CAD build for the part. Positions are in the model's coordinates, mm. Face numbers are marked on the shaded views. A direction names the side the tool comes from. Give positions to 0.01 mm unless a question says otherwise; leave off trailing zeros. Loops run counter-clockwise (first coordinate to the right, second up) from the corner with the lowest first, then second, coordinate; pieces in that order, holes last. Notation, with made-up numbers: M 72.25,47 L 88.25,47 A18 ccw 88.25,58 Z; hole C 73.25,42 d8. An arc over 180 degrees is marked long. One line per question, with ' | ' between items.
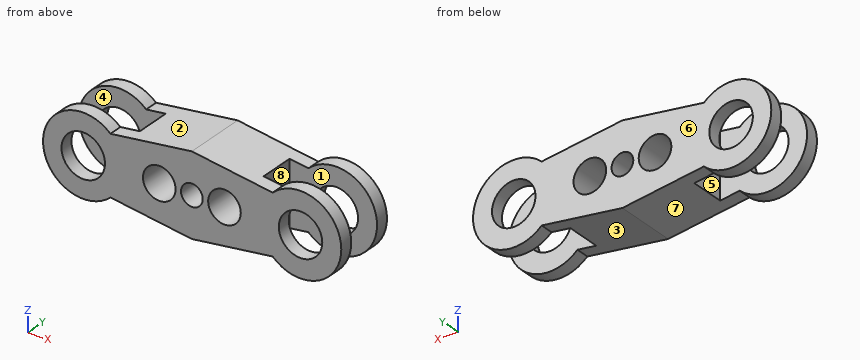
```python
from build123d import *

# Parameters (mm, degrees)
Y_KSEKLIK_EKSTR_ZYON1_OUTLINE_R   = 4
Y_KSEKLIK_EKSTR_ZYON1_OUTLINE_R_2 = 3
Y_KSEKLIK_EKSTR_ZYON1_OUTLINE_R_3 = 2
Y_KSEKLIK_EKSTR_ZYON1_DEPTH       = 11.5
KES_EKSTR_ZYON9_DEPTH             = 50
KES_EKSTR_ZYON9_DEPTH_BACK        = 50
IZIM16_W                          = 16
IZIM16_H                          = 6.5
IZIM16_W_2                        = 1.702500787


# Read off the part's stored shape, not the designer's step: Y_kseklik-Ekstr_zyon1
with BuildPart() as part:
    # Y_kseklik-Ekstr_zyon1 outline → Y_kseklik-Ekstr_zyon1 (new body)
    with BuildSketch(Plane(origin=(0, 0, 0), x_dir=(1, 0, 0), z_dir=(0, 1, 0))):
        with BuildLine():
            Line((-14.995122872, -5.45), (0, -7.5))
            Line((0, -7.5), (14.866270364, -5.46761557))
            ThreePointArc((14.866270364, -5.46761557), (27.5, 0), (14.866270364, 5.46761557))
            Line((14.866270364, 5.46761557), (0, 7.5))
            Line((0, 7.5), (-14.995122872, 5.45))
            ThreePointArc((-14.995122872, 5.45), (-27.399411806, 0), (-14.995122872, -5.45))
        make_face()
        with Locations((-20, 0)):
            Circle(Y_KSEKLIK_EKSTR_ZYON1_OUTLINE_R, mode=Mode.SUBTRACT)
        with Locations((-6, 0)):
            Circle(Y_KSEKLIK_EKSTR_ZYON1_OUTLINE_R_2, mode=Mode.SUBTRACT)
        Circle(Y_KSEKLIK_EKSTR_ZYON1_OUTLINE_R_3, mode=Mode.SUBTRACT)
        with Locations((6, 0)):
            Circle(Y_KSEKLIK_EKSTR_ZYON1_OUTLINE_R_2, mode=Mode.SUBTRACT)
        with Locations((20, 0)):
            Circle(Y_KSEKLIK_EKSTR_ZYON1_OUTLINE_R, mode=Mode.SUBTRACT)
    extrude(amount=Y_KSEKLIK_EKSTR_ZYON1_DEPTH)

    # izim16 → Kes-Ekstr_zyon9 (cut, two sides: drawn at the far end of the back side and taken through both)
    with BuildSketch(Plane.XY.offset(-KES_EKSTR_ZYON9_DEPTH_BACK)):
        with Locations((-19.399411806, 5.75)):
            Rectangle(IZIM16_W, IZIM16_H)
        with Locations((-28.2506622, 5.75)):
            Rectangle(IZIM16_W_2, IZIM16_H)
        Polygon((29.101912593, 9), (27.399411806, 9), (11.399411806, 9), (11.399411806, 2.5), (27.399411806, 2.5), (29.101912593, 2.5), align=None)
    extrude(amount=KES_EKSTR_ZYON9_DEPTH + KES_EKSTR_ZYON9_DEPTH_BACK, mode=Mode.SUBTRACT)


solid = part.part
```
Item 1: Mould opens along Y. For the marked faces 5, 6, 7 and 8 say: pulls with the +Y half, pulls with the -Y half, needs draft (parallel to the pull), parting line crosses it, or undercut.
Conclusion:
face 5: undercut | face 6: pulls with the +Y half | face 7: needs draft | face 8: undercut
Item 2: Saw through at B-B on y = 8.5. Give the cut face in (x, z), and give its area (3 significant figures).
Conclusion:
outline: M -11.4,-5.94 L 0,-7.5 L 11.4,-5.94 L 11.4,5.94 L 0,7.5 L -11.4,5.94 Z; hole C -6,0 d6; hole C 0,0 d4; hole C 6,0 d6 | area: 237 mm²
Item 3: 3-axis set-ups, long thin cutter, end or side, ignore diameter. For the marked faces 1, 2, 3 and 4: which of +Z, -Z, +X, -X, +Y, -Y reach the whole face in a straight line?
Conclusion:
face 1: +Z, -Z, +X | face 2: +Z, +Y, -Y | face 3: -Z, +Y, -Y | face 4: +Z, -Z, -X
Item 4: Drop flat-ended pins along their axis: P1, Ø6, axis at x = 8, y = 6, coming from the -Z side; P2, Ø6.5, axis at x = 0, z = 0, coming from the +Y side; P3, Ø1.5, axis at x = -19.5, y = 1.5, coming from the +Z side; P4, Ø3, axis at y = 4.5, z = 0, coming from the +X side. Give the stop position or say it passes through.
Conclusion:
P1: z = -6.82 | P2: y = 11.5 | P3: z = 7.4 | P4: x = 11.4
Item 5: Drill centre lines: line 1 along X through (y, z) = (8.5, 0); line 2 along X through (y, z) = (0.55, 0); line 3 along Y through (x, z) = (14, -2.5). Where is each one in solid material? Low to high. Write a range as [from, to].
Conclusion:
line 1: [-11.4, -9], [-3, -2], [2, 3], [9, 11.4] | line 2: [-27.4, -24], [-16, -9], [-3, -2], [2, 3], [9, 16], [24, 27.5] | line 3: [0, 2.5], [9, 11.5]
Item 6: Saw through at C-C on z = -3.5. Give the cut face in (x, y), and give its area (3 significant figures).
Conclusion:
outline: M -26.52,0 L -21.94,0 L -21.94,2.5 L -26.52,2.5 Z; M -26.52,9 L -21.94,9 L -21.94,11.5 L -26.52,11.5 Z; M -18.06,0 L 18.06,0 L 18.06,2.5 L 11.4,2.5 L 11.4,9 L 18.06,9 L 18.06,11.5 L -18.06,11.5 L -18.06,9 L -11.4,9 L -11.4,2.5 L -18.06,2.5 Z; M 21.94,0 L 26.63,0 L 26.63,2.5 L 21.94,2.5 Z; M 21.94,9 L 26.63,9 L 26.63,11.5 L 21.94,11.5 Z | area: 375 mm²
Item 7: Saw through at A-A on x = 20. Give the cut face in (y, z), and give its area (3 significant figures).
Conclusion:
outline: M 0,-7.5 L 2.5,-7.5 L 2.5,-4 L 0,-4 Z; M 0,4 L 2.5,4 L 2.5,7.5 L 0,7.5 Z; M 9,-7.5 L 11.5,-7.5 L 11.5,-4 L 9,-4 Z; M 9,4 L 11.5,4 L 11.5,7.5 L 9,7.5 Z | area: 35.0 mm²
Item 8: Saw through at D-D on y = 2. Give the cut face in (x, z).
Conclusion:
outline: M -15,-5.45 L 0,-7.5 L 14.87,-5.47 A7.5 ccw long 14.87,5.47 L 0,7.5 L -15,5.45 A7.4 ccw long Z; hole C -20,0 d8; hole C -6,0 d6; hole C 0,0 d4; hole C 6,0 d6; hole C 20,0 d8
